```python
from build123d import *

# Parameters (mm, degrees)
EXTRUDE_1_DEPTH     = 50
SKETCH_2_R          = 19
EXTRUDE_2_DEPTH     = 75
EXTRUDE_3_DEPTH     = 290
SKETCH_4_R          = 10
CUT_EXTRUDE_1_DEPTH = 170
SKETCH_5_W          = 18
SKETCH_5_H          = 18
EXTRUDE_4_DEPTH     = 19
SKETCH_7_R          = 3.25
CUT_EXTRUDE_2_DEPTH = 19
CHAMFER_1_SIZE      = 10
CHAMFER_2_SIZE      = 2


with BuildPart() as part:
    # 草图1 → 凸台-拉伸1 (new body)
    with BuildSketch(Plane(origin=(0, 0, 0), x_dir=(1, 0, 0), z_dir=(0, 1, 0))):
        with BuildLine():
            Line((-20, 27.5), (20, 27.5))
            Line((20, 27.5), (20, -27.5))
            ThreePointArc((20, -27.5), (0, -47.5), (-20, -27.5))
            Line((-20, -27.5), (-20, 27.5))
        make_face()
    extrude(amount=EXTRUDE_1_DEPTH)

    # 草图2 → 凸台-拉伸2 (add)
    with BuildSketch(Plane(origin=(0, 50, 0), x_dir=(1, 0, 0), z_dir=(0, 1, 0))):
        with Locations(Location((0, -25.772612345, 0), (0, 0, 270))):
            Circle(SKETCH_2_R)
    extrude(amount=EXTRUDE_2_DEPTH)

    # 草图3 → 凸台-拉伸3 (add)
    with BuildSketch(Plane(origin=(0, 50, 0), x_dir=(1, 0, 0), z_dir=(0, 1, 0))):
        with BuildLine():
            Line((-12.473266485, 18.913505227), (-6.7377758, 27.5))
            Line((-6.7377758, 27.5), (6.7377758, 27.5))
            Line((6.7377758, 27.5), (12.473266485, 18.913505227))
            ThreePointArc((12.473266485, 18.913505227), (0, -4.418218675), (-12.473266485, 18.913505227))
        make_face()
    extrude(amount=EXTRUDE_3_DEPTH)

    # 草图4 → 切除-拉伸1 (cut)
    with BuildSketch(Plane(origin=(0, 340, 0), x_dir=(1, 0, 0), z_dir=(0, 1, 0))):
        with Locations(Location((0, 10.581781325, 0), (0, 0, 270))):
            Circle(SKETCH_4_R)
    extrude(amount=-CUT_EXTRUDE_1_DEPTH, mode=Mode.SUBTRACT)

    # 草图5 → 凸台-拉伸4 (add)
    with BuildSketch(Plane.XZ):
        with Locations((0.33262197, -7.5)):
            Rectangle(SKETCH_5_W, SKETCH_5_H)
    extrude(amount=EXTRUDE_4_DEPTH)

    # 草图7 → 切除-拉伸2 (cut)
    with BuildSketch(Plane(origin=(9.33262197, 0, 0), x_dir=(0, 0, -1), z_dir=(1, 0, 0))):
        with Locations((7.5, -9.5)):
            Circle(SKETCH_7_R)
    extrude(amount=-CUT_EXTRUDE_2_DEPTH, mode=Mode.SUBTRACT)

    # 倒角1
    chamfer_1_edges = [part.edges().sort_by_distance(p)[0] for p in [
        (-20, 25, -27.5),
        (20, 25, -27.5),
    ]]
    chamfer(chamfer_1_edges, length=CHAMFER_1_SIZE)

    # 倒角2
    chamfer_2_edges = [part.edges().sort_by_distance(p)[0] for p in [
        (9.33262197, -9.5, -16.5),
        (9.33262197, -9.5, 1.5),
        (-8.66737803, -9.5, 1.5),
        (-8.66737803, -9.5, -16.5),
    ]]
    chamfer(chamfer_2_edges, length=CHAMFER_2_SIZE)


solid = part.part
```
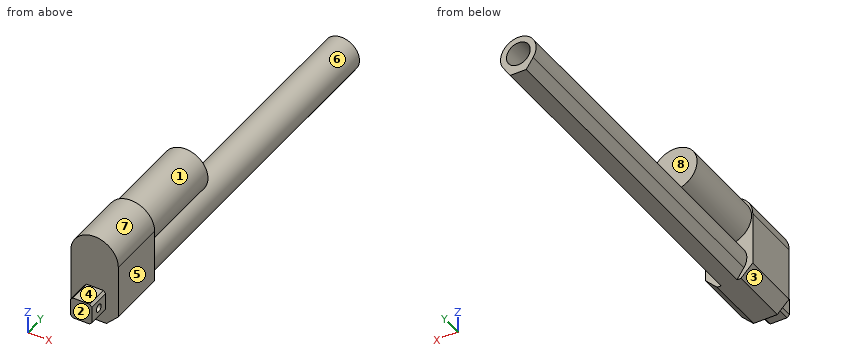
Here's how the part is built. I have some questions about the finished solid (model axes, mm). Face numbers are marked on the shaded views. A direction names the side the tool comes from. Round coordinates to 2 decimals unless told otherwise and drop trailing zeros. Loops run counter-clockwise (first coordinate to the right, second up) from the corner with the lowest first, then second, coordinate; pieces in that order, holes last. Notation, with made-up numbers: (-10.75, 89) -> (48.25, 89) arc R27 cw to (48.25, 111) -> close; hole circle Ø10 at (43, 51.25). An arc over 180 degrees is marked (long way). Answer as CSV lines item,"result". Start each with the question number.
1. If we mould it in two halves opening along Z, with no side actions, what happens to the marked faces 1, 2 and 3? For each: pulls with the +Z half, pulls with the -Z half, needs draft (parallel to the pull), parting line crosses it, or undercut.
2. For the marked faces 4, 5, 6, 7 and 8, which set-ups out of +Z, -Z, +X, -X, +Y, -Y let a thin tool reach every point of the face, with its end or its side?
3. Imagine slicing it at D-D on y = 120. Write out the boundary of the cut face in (x, z).
4. I'm going to push flat-ended pins straight in: P1, Ø1, axis at x = -0.5, y = 200, coming from the +Z side; P2, Ø4, axis at y = -8.5, z = -5, coming from the -X side; P3, Ø5, axis at x = 10, z = 17.5, coming from the -Y side. Where does each tip first touch, or does it pass through?
5. Imagine slicing it at B-B on y = 249. Write out the boundary of the cut face in (x, z).
6. I need wall thicknesses on probe 1 along Y at (x, z) = (-4.5, -7.5); probe 2 along X at (y, z) = (177, -10); probe 3 along Y at (x, z) = (-0.5, 29.5). Which ranges of each line are inside material? Lowest first, please. Write a range as from..to.
7. Imagine slicing it at C-C on z = -7.5. Write out the boundary of the cut face in (x, y).
8. Imagine slicing it at A-A on x = 0. Write out the boundary of the cut face in (y, z).
Solution:
1,face 1,"undercut"
1,face 2,"needs draft"
1,face 3,"pulls with the -Z half"
2,face 4,"+Z, +X, -X, -Y"
2,face 5,"+Z, -Z, +X, +Y, -Y"
2,face 6,"+Y"
2,face 7,"+Z, +Y, -Y"
2,face 8,"+Z, +X, -X, +Y"
3,outline,"circle Ø38 at (0, 25.77); (-12.47, -18.91) -> (-6.74, -27.5) -> (6.74, -27.5) -> (12.47, -18.91) arc R15 ccw (long way) to start"
4,P1,"z = 4.42"
4,P2,"x = -8.67"
4,P3,"y = 0"
5,outline,"(-12.47, -18.91) -> (-6.74, -27.5) -> (6.74, -27.5) -> (12.47, -18.91) arc R15 ccw (long way) to start; hole circle Ø20 at (0, -10.58)"
6,probe 1,"-19..-12.75, -6.25..170"
6,probe 2,"-14.99..-9.98, 9.98..14.99"
6,probe 3,"0..125"
7,outline,"(-20, 0) -> (-8.67, 0) -> (-8.67, -6.25) -> (9.33, -6.25) -> (9.33, 0) -> (20, 0) -> (20, 50) -> (14.68, 50) -> (14.68, 340) -> (9.51, 340) -> (9.51, 170) -> (-9.51, 170) -> (-9.51, 340) -> (-14.68, 340) -> (-14.68, 50) -> (-20, 50) -> close; (-8.67, -19) -> (9.33, -19) -> (9.33, -12.75) -> (-8.67, -12.75) -> close"
8,outline,"(-19, -16.5) -> (0, -16.5) -> (0, -27.5) -> (340, -27.5) -> (340, -20.58) -> (170, -20.58) -> (170, -0.58) -> (340, -0.58) -> (340, 4.42) -> (50, 4.42) -> (50, 6.77) -> (125, 6.77) -> (125, 44.77) -> (50, 44.77) -> (50, 47.5) -> (0, 47.5) -> (0, 1.5) -> (-19, 1.5) -> close; hole circle Ø6.5 at (-9.5, -7.5)"
